Could you check a few things on this model? Use its own coordinates, in mm. Give positions to 0.01 mm unless a question says otherwise; leave off trailing zeros. Loops run counter-clockwise (first coordinate to the right, second up) from the corner with the lowest first, then second, coordinate; pieces in that order, holes last. Notation, with made-up numbers: M 48.25,76.5 L 70.25,76.5 A12 ccw 70.25,83.5 Z; hole C 30.25,-39 d2. An arc over 180 degrees is marked long. Use CSV: the item, a comma, the result in double quotes.
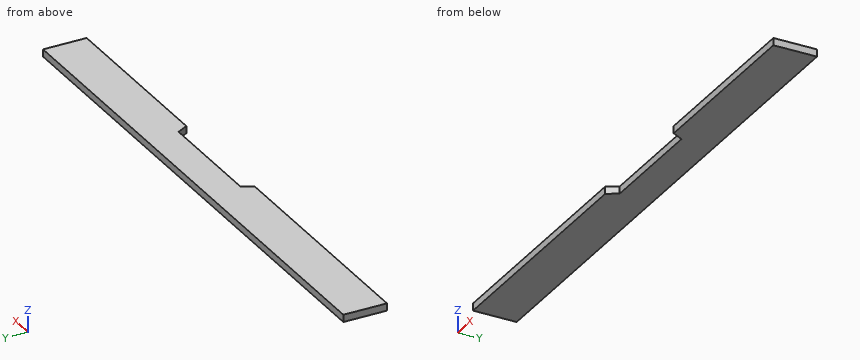
```python
from build123d import *

# Parameters (mm, degrees)
SKETCH1_W           = 120.65
SKETCH1_H           = 9.525
BOSS_EXTRUDE1_DEPTH = 0.79375
CUT_EXTRUDE1_DEPTH  = 2.5875


with BuildPart() as part:
    # Sketch1 → Boss-Extrude1 (new body, symmetric)
    with BuildSketch(Plane.XY):
        Rectangle(SKETCH1_W, SKETCH1_H)
    extrude(amount=BOSS_EXTRUDE1_DEPTH, both=True)

    # Sketch2 → Cut-Extrude1 (cut, through all)
    with BuildSketch(Plane.XY.offset(0.79375)):
        Polygon((-7.202243564, -4.7625), (-5.855664106, -2.3495), (18.960360816, -2.3495), (20.306940273, -4.7625), align=None)
    extrude(amount=-CUT_EXTRUDE1_DEPTH, mode=Mode.SUBTRACT)


solid = part.part
```
1. I want a section at A-A, the plane z = -0.2. List the corners of the cut face in (x, y) for me (1 decimal), then the cut area to 3 significant figures.
Outcome:
outline,"M -60.3,-4.8 L -7.2,-4.8 L -5.9,-2.3 L 19,-2.3 L 20.3,-4.8 L 60.3,-4.8 L 60.3,4.8 L -60.3,4.8 Z"
area,"1,090 mm2"
2. I want a section at B-B, the plane y = -3.75. List the corners of the cut face in (x, z) for me (3 decimals).
Outcome:
outline,"M -60.325,-0.794 L -6.637,-0.794 L -6.637,0.794 L -60.325,0.794 Z; M 19.742,-0.794 L 60.325,-0.794 L 60.325,0.794 L 19.742,0.794 Z"
3. Please list where these lines run through material, in increasing order: line 1 (Y direction, x = 0, z = -0.25); line 2 (X direction, y = -3.5, z = 0.3) (3 decimals); line 3 (X direction, y = -4, z = -0.5) (3 decimals).
Outcome:
line 1,"-2.35 to 4.76"
line 2,"-60.325 to -6.498, 19.602 to 60.325"
line 3,"-60.325 to -6.777, 19.881 to 60.325"
